Can you work these out from the model? Positions are in its coordinate system, mm. Face numbers are marked on the shaded views. A direction names the side the tool comes from. Give positions to 0.01 mm unless a question says otherwise; leave off trailing zeros. Order: outer loops, then holes, each group sorted by start corner. A loop starts at its lowest first (then second) coordinate and runs counter-clockwise, first axis right, second up. Notation, with made-up numbers: (48, 78) -> (95, 78) arc R17 ccw to (95, 85) -> close; hole circle Ø6 at (-28, -4). An arc over 180 degrees is marked (long way). Answer as CSV lines item,"result".
```python
from build123d import *
from build123d.topology import SkipClean

# Parameters (mm, degrees)
SALIENTE_EXTRUIR1_DEPTH    = 2.4
CORTAR_EXTRUIR1_DEPTH      = 26.29347742
CORTAR_EXTRUIR1_DEPTH_BACK = 26.29347742
CROQUIS2_R                 = 1.5
CROQUIS3_R                 = 1.5
SALIENTE_EXTRUIR2_DEPTH    = 7.5
CORTAR_EXTRUIR2_DEPTH      = 3.1
REDONDEO1_R                = 2
REDONDEO2_R                = 1


with BuildPart() as part:
    # Croquis1 → Saliente-Extruir1 (new, symmetric)
    with BuildSketch(Plane(origin=(0, 0, 0), x_dir=(0, 0, -1), z_dir=(1, 0, 0))):
        with BuildLine():
            Line((-24, 3), (24, 3))
            ThreePointArc((24, 3), (24.707106781, 2.707106781), (25, 2))
            Line((25, 2), (25, -2))
            ThreePointArc((25, -2), (24.707106781, -2.707106781), (24, -3))
            Line((24, -3), (-24, -3))
            ThreePointArc((-24, -3), (-24.707106781, -2.707106781), (-25, -2))
            Line((-25, -2), (-25, 2))
            ThreePointArc((-25, 2), (-24.707106781, 2.707106781), (-24, 3))
        make_face()
    extrude(amount=SALIENTE_EXTRUIR1_DEPTH, both=True)

    # Croquis2 → Cortar-Extruir1 (cut, two sides: drawn at the far end of the back side and taken through both)
    with BuildSketch(Plane(origin=(0, 0, 0), x_dir=(0, 0, -1), z_dir=(1, 0, 0)).offset(-CORTAR_EXTRUIR1_DEPTH_BACK)):
        with Locations((-21, 0)):
            Circle(CROQUIS2_R)
        with Locations((21, 0)):
            Circle(CROQUIS2_R)
    extrude(amount=CORTAR_EXTRUIR1_DEPTH + CORTAR_EXTRUIR1_DEPTH_BACK, mode=Mode.SUBTRACT)

    # Croquis3 → Saliente-Extruir2 (add, symmetric)
    with SkipClean():  # the faces are left unmerged after this step: merging them gives an invalid solid
        with BuildSketch(Plane(origin=(0, 0, 0), x_dir=(0, 0, -1), z_dir=(1, 0, 0))):
            with BuildLine():
                Line((-25, 2), (-25, -2))
                ThreePointArc((-25, -2), (-24.707106781, -2.707106781), (-24, -3))
                Line((-24, -3), (-10, -3))
                Line((-10, -3), (-10, 3))
                Line((-10, 3), (-24, 3))
                ThreePointArc((-24, 3), (-24.707106781, 2.707106781), (-25, 2))
            make_face()
            with Locations((-21, 0)):
                Circle(CROQUIS3_R, mode=Mode.SUBTRACT)
        extrude(amount=SALIENTE_EXTRUIR2_DEPTH, both=True)
    add(part.part.scale(1), mode=Mode.REPLACE)  # the faces are merged on a copy

    # Croquis4 → Cortar-Extruir2 (cut, symmetric)
    with BuildSketch(Plane(origin=(0, 0, 0), x_dir=(0, 0, -1), z_dir=(1, 0, 0))):
        with BuildLine():
            Line((-24, 3), (-15, 3))
            Line((-15, 3), (-15, -3))
            Line((-15, -3), (-24, -3))
            ThreePointArc((-24, -3), (-24.707106781, -2.707106781), (-25, -2))
            Line((-25, -2), (-25, 2))
            ThreePointArc((-25, 2), (-24.707106781, 2.707106781), (-24, 3))
        make_face()
    extrude(amount=CORTAR_EXTRUIR2_DEPTH, both=True, mode=Mode.SUBTRACT)

    # Redondeo1
    redondeo1_edges = [part.edges().sort_by_distance(p)[0] for p in [
        (-2.4, 0, 10),
        (2.4, 0, 10),
        (-7.5, 0, 10),
        (7.5, 0, 10),
    ]]
    fillet(redondeo1_edges, radius=REDONDEO1_R)

    # Redondeo2
    redondeo2_edges = [part.edges().sort_by_distance(p)[0] for p in [
        (3.1, 0, 15),
        (-3.1, 0, 15),
    ]]
    fillet(redondeo2_edges, radius=REDONDEO2_R)


solid = part.part
```
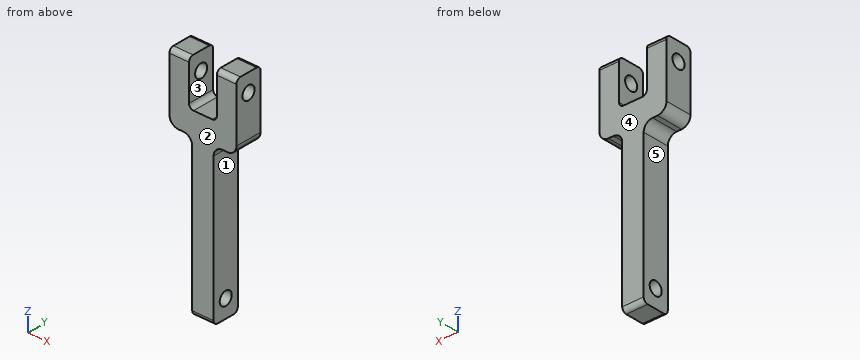
Item 1: We'd pull the mould along X, two halves only. Please class the marked faces 3, 4 and 5: released by +X, released by -X, zero draft, split by the parting line, or undercut.
Numbers:
face 3,"undercut"
face 4,"zero draft"
face 5,"released by -X"
Item 2: Imagine slicing it at D-D, the plane z = -21. Please give me the cut outline in (x, y), then the cut area to 3 significant figures.
Numbers:
outline,"(-2.4, -3) -> (2.4, -3) -> (2.4, -1.5) -> (-2.4, -1.5) -> close; (-2.4, 1.5) -> (2.4, 1.5) -> (2.4, 3) -> (-2.4, 3) -> close"
area,"14.4 mm²"
Item 3: Imagine slicing it at B-B, the plane y = 0. Give the number of separate pieces and of enclosed holes in the cut face, then the cut area to 3 significant figures.
Numbers:
separate pieces,"4"
enclosed holes,"0"
area,"291 mm²"
Item 4: Imagine slicing it at C-C, the plane x = 1.25. Please give me the cut outline in (y, z).
Numbers:
outline,"(-3, -24) arc R1 ccw to (-2, -25) -> (2, -25) arc R1 ccw to (3, -24) -> (3, 15) -> (-3, 15) -> close; hole circle Ø3 at (0, -21)"
Item 5: For the marked faces 1 and 2, which set-ups out of +Z, -Z, +X, -X, +Y, -Y let a thin tool reach every point of the face, with its end or its side?
Numbers:
face 1,"-Z, +X, +Y, -Y"
face 2,"+Z, -Z, +X, -X, -Y"
Item 6: Please list where these lines run through material, in increasing order: line 1 along X through (y, z) = (1.55, 22.5); line 2 along Y through (x, z) = (-6.55, 21); line 3 along X through (y, z) = (0.15, -17).
Numbers:
line 1,"x = -7.5 to -3.1, 3.1 to 7.5"
line 2,"y = -3 to -1.5, 1.5 to 3"
line 3,"x = -2.4 to 2.4"
Item 7: Imagine slicing it at A-A, the plane z = 21. Please give me the cut outline in (x, y).
Numbers:
outline,"(-7.5, -3) -> (-3.1, -3) -> (-3.1, -1.5) -> (-7.5, -1.5) -> close; (-7.5, 1.5) -> (-3.1, 1.5) -> (-3.1, 3) -> (-7.5, 3) -> close; (3.1, -3) -> (7.5, -3) -> (7.5, -1.5) -> (3.1, -1.5) -> close; (3.1, 1.5) -> (7.5, 1.5) -> (7.5, 3) -> (3.1, 3) -> close"
Item 8: For pin 1 (3.5 mm diameter, centred on y = 0, z = 21, fed in from +X); pin 2 (0.9 mm diameter, centred on x = 4.5, y = 1, fed in from -Z); pin 3 (1.8 mm diameter, centred on y = 0, z = -14.5, fed in from -X); pin 4 (1 mm diameter, centred on y = 2.5, z = 2, fed in from +X), each with a flat end and sliding along its axis, tell me the tip position at first contact or that it passes through.
Numbers:
pin 1,"stops at x = 7.5"
pin 2,"stops at z = 9.97"
pin 3,"stops at x = -2.4"
pin 4,"stops at x = 2.4"
